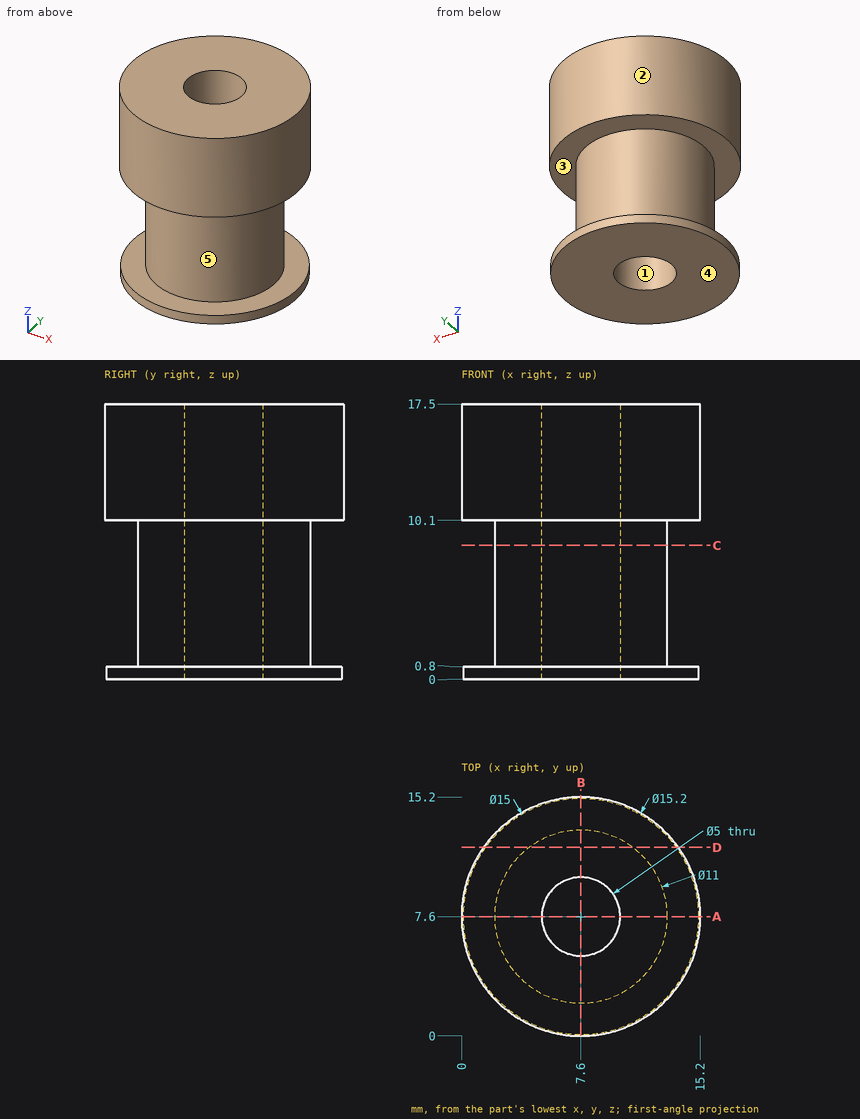
Source: three-view drawing plus pictorial views. Frame: mm from the lowest corner of the part. A direction names the side the tool comes from. Give positions to 0.01 mm unless a question says otherwise; leave off trailing zeros. Order: outer loops, then holes, each group sorted by start corner. A loop starts at its lowest first (then second) coordinate and runs counter-clockwise, first axis right, second up. Notation, with made-up numbers: (31, -24.75) -> (52, -24.75) arc R34 cw to (52, 13.25) -> close; hole circle Ø8 at (-15, 88.5). An arc over 180 degrees is marked (long way). Use a Markdown table: item, result.
Q1. Section A-A (y = 7.6). Return the cut outline in (x, z).
A:
| item | result |
|---|---|
| outline | (0, 10.1) -> (2.1, 10.1) -> (2.1, 0.8) -> (0.1, 0.8) -> (0.1, 0) -> (5.1, 0) -> (5.1, 17.5) -> (0, 17.5) -> close; (10.1, 0) -> (15.1, 0) -> (15.1, 0.8) -> (13.1, 0.8) -> (13.1, 10.1) -> (15.2, 10.1) -> (15.2, 17.5) -> (10.1, 17.5) -> close |
Q2. Section C-C (z = 8.5). Return the cut outline in (x, y).
A:
| item | result |
|---|---|
| outline | circle Ø11 at (7.6, 7.6); hole circle Ø5 at (7.6, 7.6) |
Q3. Section D-D (y = 12). Return the cut outline in (x, z).
A:
| item | result |
|---|---|
| outline | (1.4, 10.1) -> (4.3, 10.1) -> (4.3, 0.8) -> (1.53, 0.8) -> (1.53, 0) -> (13.67, 0) -> (13.67, 0.8) -> (10.9, 0.8) -> (10.9, 10.1) -> (13.8, 10.1) -> (13.8, 17.5) -> (1.4, 17.5) -> close |
Q4. Access query for the marked faces 4 and 5. Directions: +Z, -Z, +X, -X, +Y, -Y. A direction counts if a zero-diameter tool reaches every point of the face in a straight line with its end or side. Return the directions, or none.
A:
| item | result |
|---|---|
| face 4 | -Z, +X, -X, +Y, -Y |
| face 5 | none |
Q5. First-contact query: P1, Ø6, axis at y = 8, z = 5.5, coming from the -X side; P2, Ø8, axis at y = 4, z = 2.5, coming from the +X side; P3, Ø3, axis at x = 4.5, y = 7, coming from the -Z side; P4, Ø4, axis at x = 10.5, z = 11, coming from the +Y side. Flat tips, straight axial feed; report the tip coordinate or a pass-through.
A:
| item | result |
|---|---|
| P1 | x = 2.1 |
| P2 | x = 15.1 |
| P3 | z = 0 |
| P4 | y = 15.15 |
Q6. Material intervals for line 1 (Y direction, x = 7.6, z = 9); line 2 (Z direction, x = 1.5, y = 9.75); line 3 (Y direction, x = 7.6, z = 11.75), sorted ascending. Write a range as [from, to].
A:
| item | result |
|---|---|
| line 1 | [2.1, 5.1], [10.1, 13.1] |
| line 2 | [0, 0.8], [10.1, 17.5] |
| line 3 | [0, 5.1], [10.1, 15.2] |
Q7. Pull-direction query (X, two-part tool) for the marked faces 1, 2 and 3; classes: +X half, -X half, draft (parallel to the pull), parting line (faces both ways), or undercut.
A:
| item | result |
|---|---|
| face 1 | undercut |
| face 2 | parting line |
| face 3 | draft |
